from build123d import *

# Parameters (mm, degrees)
SKETCH2_R           = 175
BOSS_EXTRUDE1_DEPTH = 30
SKETCH3_R           = 50
BOSS_EXTRUDE2_DEPTH = 1110
SKETCH7_W           = 2450
SKETCH7_H           = 1
BOSS_EXTRUDE3_DEPTH = 1060
SKETCH8_W           = 2450
SKETCH8_H           = 4
BOSS_EXTRUDE4_DEPTH = 80
SKETCH11_W          = 2450
SKETCH11_H          = 4.938385514
BOSS_EXTRUDE5_DEPTH = 80
SKETCH12_R          = 50
BOSS_EXTRUDE6_DEPTH = 20


with BuildPart() as part:
    # Sketch2 → Boss-Extrude1 (new body)
    with BuildSketch(Plane(origin=(0, 0, 0), x_dir=(1, 0, 0), z_dir=(0, 1, 0))):
        with Locations(Location((0, 0, 0), (0, 0, 270))):
            Circle(SKETCH2_R)
    extrude(amount=BOSS_EXTRUDE1_DEPTH)

    # Sketch3 → Boss-Extrude2 (add)
    with BuildSketch(Plane(origin=(0, 30, 0), x_dir=(1, 0, 0), z_dir=(0, 1, 0))):
        with Locations(Location((0, 0, 0), (0, 0, 270))):
            Circle(SKETCH3_R)
    extrude(amount=BOSS_EXTRUDE2_DEPTH)

    # Sketch7 → Boss-Extrude3 (add)
    with BuildSketch(Plane(origin=(0, 1140, 0), x_dir=(1, 0, 0), z_dir=(0, 1, 0))):
        with Locations((1225, 0)):
            Rectangle(SKETCH7_W, SKETCH7_H)
    extrude(amount=-BOSS_EXTRUDE3_DEPTH)

    # Sketch8 → Boss-Extrude4 (add)
    with BuildSketch(Plane(origin=(0, 1140, 0), x_dir=(1, 0, 0), z_dir=(0, 1, 0))):
        with Locations((1225, 0)):
            Rectangle(SKETCH8_W, SKETCH8_H)
    extrude(amount=-BOSS_EXTRUDE4_DEPTH)

    # Sketch11 → Boss-Extrude5 (add)
    with BuildSketch(Plane(origin=(0, 80, 0), x_dir=(-1, 0, 0), z_dir=(0, -1, 0))):
        with Locations((-1225, 0)):
            Rectangle(SKETCH11_W, SKETCH11_H)
    extrude(amount=-BOSS_EXTRUDE5_DEPTH)

    # Sketch12 → Boss-Extrude6 (add)
    with BuildSketch(Plane(origin=(0, 1140, 0), x_dir=(1, 0, 0), z_dir=(0, 1, 0))):
        with Locations(Location((0, 0, 0), (0, 0, 270))):
            Circle(SKETCH12_R)
    extrude(amount=BOSS_EXTRUDE6_DEPTH)


solid = part.part
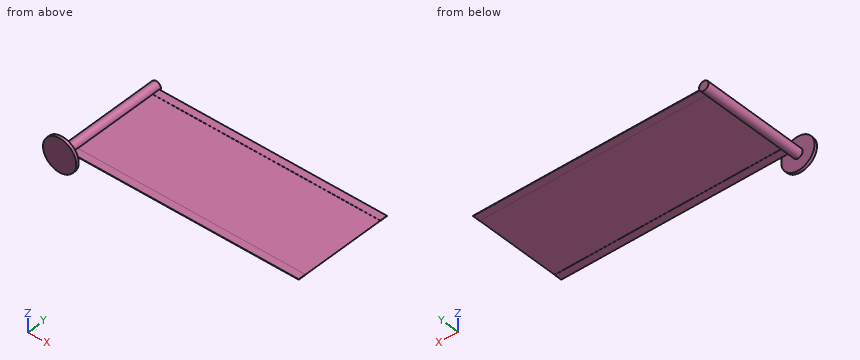
The listing builds one solid part. Answer for the finished solid, in the listing's coordinates (mm). Round coordinates to 2 decimals unless told otherwise and drop trailing zeros. Write each loop counter-clockwise with the first axis right and the second up, starting at its lowest first coordinate (ties: lowest second). Pieces come first, ordered by that corner, then holes. Notation, with made-up numbers: M -19,-17 L 27,-17 A26 ccw 27,16 Z; hole C -30.75,86.25 d8. An arc over 180 degrees is marked long. Write each question's results on one line, items separated by ' | '. Start each with the question number.
(1) The part is cut by section A-A, the plane x = 664.5. Write down the section's boundary in (y, z), and give its area (3 significant figures).
(2) The part is cut by section C-C, the plane x = 0. Write down the section's boundary in (y, z), and give its area (4 significant figures).
(3) Each of these flat-tipped pins is pushed along its axis until it touches: P1, Ø10, axis at x = 1021.5, y = 520.5, coming from the +Z side; P2, Ø4, axis at x = 1509.5, z = 0.5, coming from the -Y side; P3, Ø1.5, axis at x = 1959.5, y = 379, coming from the -Z side. Where does it stop, or does it pass through?
(4) The part is cut by section B-B, the plane y = 498. Write down the section's boundary in (x, z).
(5) Find the intervals of material crossed by line 1 (Z direction, x = 442, y = 465); line 2 (Y direction, x = 39.5, z = 122.5); line 3 (X direction, y = 563, z = -1.5), in increasing order.
(6) The part is cut by section D-D, the plane z = -93. Write down the section's boundary in (x, y).
Worked answers:
1) outline: M 80,-2.47 L 160,-2.47 L 160,-0.5 L 1060,-0.5 L 1060,-2 L 1140,-2 L 1140,2 L 1060,2 L 1060,0.5 L 160,0.5 L 160,2.47 L 80,2.47 Z | area: 1,620 mm²
2) outline: M 0,-175 L 30,-175 L 30,-50 L 1160,-50 L 1160,50 L 30,50 L 30,175 L 0,175 Z | area: 123,500 mm²
3) P1: stops at z = 0.5 | P2: stops at y = 80 | P3: stops at z = -0.5
4) outline: M 50,-0.5 L 2450,-0.5 L 2450,0.5 L 50,0.5 A50 ccw long Z
5) line 1: z = -0.5 to 0.5 | line 2: y = 0 to 30 | line 3: x = -49.98 to 49.98
6) outline: M -148.24,0 L 148.24,0 L 148.24,30 L -148.24,30 Z
